```python
from build123d import *

# Parameters (mm, degrees)
F0_W           = 65
F0_H           = 80
F1_DEPTH       = 10
F3_D           = 5
F3_CSINK_D     = 10
F3_CSINK_ANGLE = 90
F5_W           = 6
F5_H           = 25
F4_R           = 3
F7_DEPTH       = 10
F6_W           = 6
F6_H           = 25
F8_DEPTH       = 10
F9_R           = 3
F10_DEPTH      = 25


with BuildPart() as f1:
    # F0 (on Front) → F1 (new body)
    with BuildSketch(Plane.XZ):
        Rectangle(F0_W, F0_H)
    extrude(amount=F1_DEPTH)

    # F3 (through all)
    with Locations(Plane(origin=(0, 0, 0), x_dir=(1, 0, 0), z_dir=(0, 1, 0))):
        with Locations((-20, 10), (20, 10)):
            CounterSinkHole(F3_D / 2, F3_CSINK_D / 2, counter_sink_angle=F3_CSINK_ANGLE)

    # F5 (on Front) + F4 (on Front) → F7 (cut)
    with BuildSketch(Plane.XZ):
        with Locations((-25, 27.5)):
            Rectangle(F5_W, F5_H)
    with BuildSketch(Plane.XZ):
        with Locations((-25, 15)):
            Circle(F4_R)
    extrude(amount=F7_DEPTH, mode=Mode.SUBTRACT)

    # F6 (on Front) → F8 (cut)
    with BuildSketch(Plane.XZ):
        with Locations((25, 27.5)):
            Rectangle(F6_W, F6_H)
    extrude(amount=F8_DEPTH, mode=Mode.SUBTRACT)

    # F9 (on Front) → F10 (cut)
    with BuildSketch(Plane.XZ):
        with Locations((25, 15)):
            Circle(F9_R)
    extrude(amount=F10_DEPTH, mode=Mode.SUBTRACT)


solid = f1.part
```
Here's how the part is built. I have some questions about the finished solid (model axes, mm). A direction names the side the tool comes from. Give positions to 0.01 mm unless a question says otherwise; leave off trailing zeros. Loops run counter-clockwise (first coordinate to the right, second up) from the corner with the lowest first, then second, coordinate; pieces in that order, holes last. Notation, with made-up numbers: M -23,-17.75 L -17,-17.75 A7 ccw -17,-4.75 Z; hole C -10,6.25 d1. An arc over 180 degrees is marked long. Use one line per item in the form item = value. Start each with the question number.
Q1. I need wall thicknesses on line 1 along X through (y, z) = (-6, -10); line 2 along X through (y, z) = (-2, 24); line 3 along Z through (x, y) = (-20, -7.5). Which ranges of each line are inside material? Lowest first, please.
Q2. If we section it at A-A (x = -20): Write out the boundary of the cut face in (y, z).
Q3. Will this pin go through, and if not, where does the flat tip stop? pin 1 Ø6 at (x, z) = (-20, -10) entering from +Y.
Q4. If we section it at C-C (z = 30): Write out the boundary of the cut face in (x, y), then the cut area to 3 significant figures.
Q5. If we section it at D-D (y = -1): Write out the boundary of the cut face in (x, z).
Q6. Thinking about a two-plate mould opening in X: for faces 1 (the flat face through (22, -5, 27)), 2 (the cylindrical face through (-25, -5, 12)), 3 (the flat face through (32.5, -5, -1)), 4 (the flat face through (0, -10, 1)), which applies, +X half, -X half, draft (parallel to the pull), parting line (faces both ways), or undercut?
Q7. If we section it at B-B (y = -6.75): Write out the boundary of the cut face in (x, z), then the cut area to 3 significant figures.
Q8. Which directions (+Z, -Z, +X, -X, +Y, -Y) give clear straight access to the entire face, cutting with the end or side of a thin tool? Please do faces 5 (the flat face through (0, 0, 1)), 6 (the flat face through (-28, -5, 27)).
Taken from the geometry:
q1.line_1 = -32.5 to -22.5, -17.5 to 17.5, 22.5 to 32.5
q1.line_2 = -32.5 to -28, -22 to 22, 28 to 32.5
q1.line_3 = -40 to -12.5, -7.5 to 40
q2.outline = M -10,-40 L 0,-40 L 0,-15 L -2.5,-12.5 L -10,-12.5 Z; M -10,-7.5 L -2.5,-7.5 L 0,-5 L 0,40 L -10,40 Z
q3.pin_1 = -2
q4.outline = M -32.5,-10 L -28,-10 L -28,0 L -32.5,0 Z; M -22,-10 L 22,-10 L 22,0 L -22,0 Z; M 28,-10 L 32.5,-10 L 32.5,0 L 28,0 Z
q4.area = 530 mm^2
q5.outline = M -32.5,-40 L 32.5,-40 L 32.5,40 L 28,40 L 28,15 A3 cw 22,15 L 22,40 L -22,40 L -22,15 A3 cw -28,15 L -28,40 L -32.5,40 Z; hole C -20,-10 d8; hole C 20,-10 d8
q6.face_1 = undercut
q6.face_2 = undercut
q6.face_3 = +X half
q6.face_4 = draft
q7.outline = M -32.5,-40 L 32.5,-40 L 32.5,40 L 28,40 L 28,15 A3 cw 22,15 L 22,40 L -22,40 L -22,15 A3 cw -28,15 L -28,40 L -32.5,40 Z; hole C -20,-10 d5; hole C 20,-10 d5
q7.area = 4,830 mm^2
q8.face_5 = +Z, -Z, +X, -X, +Y
q8.face_6 = +Z, +Y, -Y
